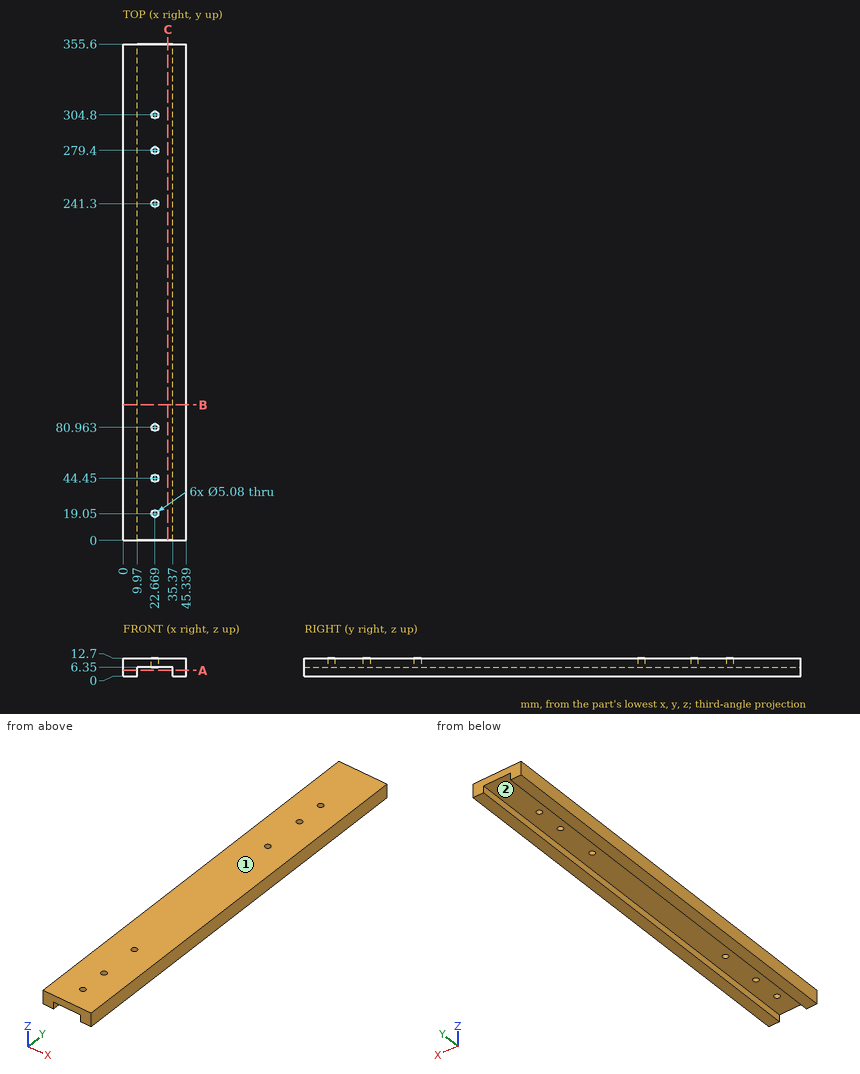
Input: dimensioned drawing with shaded views. Units: mm. Origin: part minimum x, y, z. Give positions to 0.01 mm unless a question says otherwise; leave off trailing zeros. Write each loop counter-clockwise with the first axis right and the second up, starting at its lowest first coordinate (ties: lowest second). Pieces come first, ordered by that corner, then holes.
Q1. First-contact query: P1, Ø20.5, axis at x = 22.5, y = 129, coming from the -Z side; P2, Ø4, axis at x = 12.5, z = 2, coming from the -Y side. Flat tips, straight axial feed; report the tip coordinate or a pass-through.
Q2. Section C-C, the plane x = 32. Output: boundary loops of the cut face in (y, z), plus the area to 3 significant figures.
Q3. Material intervals for probe 1 along X at (y, z) = (259.5, 6); probe 2 along X at (y, z) = (241.3, 10.25); probe 3 along Z at (x, y) = (18, 218.5), sorted ascending.
Q4. Section A-A, the plane z = 4. Output: boundary loops of the cut face in (x, y).
Q5. Pull-direction query (X, two-part tool) for the marked faces 1 and 2; classes: pulls with the +X half, pulls with the -X half, needs draft (parallel to the pull), parting line crosses it, or undercut.
Q6. Section B-B, the plane y = 97. Output: boundary loops of the cut face in (x, z).
Filled in:
1. P1: stops at z = 6.35
1. P2: passes through
2. outline: (0, 6.35) - (355.6, 6.35) - (355.6, 12.7) - (0, 12.7) - close
2. area: 2,260 mm2
3. probe 1: x = 0 to 9.97, 35.37 to 45.34
3. probe 2: x = 0 to 20.13, 25.21 to 45.34
3. probe 3: z = 6.35 to 12.7
4. outline: (0, 0) - (9.97, 0) - (9.97, 355.6) - (0, 355.6) - close; (35.37, 0) - (45.34, 0) - (45.34, 355.6) - (35.37, 355.6) - close
5. face 1: needs draft
5. face 2: undercut
6. outline: (0, 0) - (9.97, 0) - (9.97, 6.35) - (35.37, 6.35) - (35.37, 0) - (45.34, 0) - (45.34, 12.7) - (0, 12.7) - close
